Read the model definition and answer for the solid it produces. Units are mm, in the model's axes. Give positions to 0.01 mm unless a question says otherwise; leave off trailing zeros. Order: outer loops, then holes, each group sorted by start corner. A loop starts at its lowest first (then second) coordinate and runs counter-clockwise, first axis right, second up. Notation, with made-up numbers: (60.5, 83) -> (82.5, 83) arc R22 ccw to (82.5, 122) -> close; hole circle Ø6 at (81, 11). An arc over 180 degrees is marked (long way). Answer as CSV lines item,"result". Start each with the question number.
1) Find section C-C (y = -0.25). Determine the outline of the cut face in (x, z), and give its area (3 significant figures).
2) A flat-ended cylindrical pin translates along its axis: pin 1 Ø3 at (x, z) = (0.5, -20.5) entering from +Y. Find the tip coordinate at first contact, or state that the pin passes through.
3) Find section A-A (x = -17). Determine the outline of the cut face in (y, z).
4) Straight lines are drawn through the part: L1, parallel to Z at x = -3, y = -0.5; L2, parallel to Z at x = -24, y = -0.25; L3, parallel to Z at x = 2.5, y = -0.3. For each, find the intervals that lie inside material, in ascending order. Write a range as from..to.
5) Find section B-B (z = -40). Determine the outline of the cut face in (x, y), and give its area (3 significant figures).
```python
from build123d import *

# Parameters (mm, degrees)
F1_DEPTH = 0.55
F2_W     = 52
F2_H     = 40
F3_DEPTH = 0.551
F5_DEPTH = 0.551


with BuildPart() as f1:
    # F0 (on Front) → F1 (new body)
    with BuildSketch(Plane.XZ):
        with BuildLine():
            ThreePointArc((55, 63), (51.485281, 71.485281), (43, 75))
            Line((43, 75), (-43, 75))
            ThreePointArc((-43, 75), (-51.485281, 71.485281), (-55, 63))
            Line((-55, 63), (-55, -63))
            ThreePointArc((-55, -63), (-51.485281, -71.485281), (-43, -75))
            Line((-43, -75), (43, -75))
            ThreePointArc((43, -75), (51.485281, -71.485281), (55, -63))
            Line((55, -63), (55, 63))
        make_face()
    extrude(amount=F1_DEPTH)

    # F2 (on Front) → F3 (cut, through all)
    with BuildSketch(Plane.XZ):
        with BuildLine():
            Line((0, 4), (-8, 4))
            ThreePointArc((-8, 4), (-8.953329, -5.646755), (-11.5, -15))
            ThreePointArc((-11.5, -15), (-5.917981, -17.089922), (0, -17.8))
            ThreePointArc((0, -17.8), (5.917981, -17.089922), (11.5, -15))
            ThreePointArc((11.5, -15), (8.953329, -5.646755), (8, 4))
            Line((8, 4), (0, 4))
        make_face()
        with Locations((0, -45)):
            Rectangle(F2_W, F2_H)
    extrude(amount=F3_DEPTH, mode=Mode.SUBTRACT)

    # F4 (on Front) → F5 (cut, through all)
    with BuildSketch(Plane.XZ):
        with BuildLine():
            Line((-8, 61), (8, 61))
            ThreePointArc((8, 61), (10.471386, 63.122839), (8.745688, 65.8862))
            Line((8.745688, 65.8862), (0.745688, 68.3862))
            ThreePointArc((0.745688, 68.3862), (0, 68.5), (-0.745687, 68.3862))
            Line((-0.745687, 68.3862), (-8.745687, 65.8862))
            ThreePointArc((-8.745687, 65.8862), (-10.471386, 63.122839), (-8, 61))
        make_face()
    extrude(amount=F5_DEPTH, mode=Mode.SUBTRACT)


solid = f1.part
```
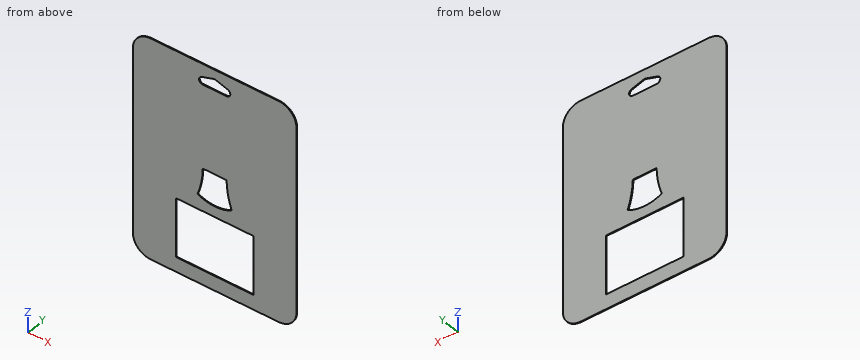
Findings below:
1,outline,"(-55, -63) arc R12 ccw to (-43, -75) -> (43, -75) arc R12 ccw to (55, -63) -> (55, 63) arc R12 ccw to (43, 75) -> (-43, 75) arc R12 ccw to (-55, 63) -> close; hole (-26, -65) -> (26, -65) -> (26, -25) -> (-26, -25) -> close; hole (-11.5, -15) arc R25.02 ccw to (0, -17.8) arc R25.02 ccw to (11.5, -15) arc R58 cw to (8, 4) -> (-8, 4) arc R58 cw to start; hole (-8.75, 65.89) arc R2.5 ccw to (-8, 61) -> (8, 61) arc R2.5 ccw to (8.75, 65.89) -> (0.75, 68.39) arc R2.5 ccw to (-0.75, 68.39) -> close"
1,area,"13,800 mm²"
2,pin 1,"y = 0"
3,outline,"(-0.55, -75) -> (0, -75) -> (0, -65) -> (-0.55, -65) -> close; (-0.55, -25) -> (0, -25) -> (0, 75) -> (-0.55, 75) -> close"
4,L1,"-75..-65, -25..-17.62, 4..61, 67.68..75"
4,L2,"-75..-65, -25..75"
4,L3,"-75..-65, -25..-17.67, 4..61, 67.84..75"
5,outline,"(-55, -0.55) -> (-26, -0.55) -> (-26, 0) -> (-55, 0) -> close; (26, -0.55) -> (55, -0.55) -> (55, 0) -> (26, 0) -> close"
5,area,"31.9 mm²"
